```python
from build123d import *

# Parameters (mm, degrees)
BOSS_EXTRUDE1_DEPTH       = 45
M6X1_0_TAPPED_HOLE1_D     = 5
M6X1_0_TAPPED_HOLE1_DEPTH = 10
M6X1_0_TAPPED_HOLE1_TIP   = 1.502151548
SKETCH5_R                 = 12.5
SKETCH5_R_2               = 14.5
CUT_EXTRUDE1_DEPTH        = 10
SKETCH6_R                 = 14.5
CUT_EXTRUDE2_DEPTH        = 3
CUT_EXTRUDE3_DEPTH        = 86.755466298
CUT_EXTRUDE3_DEPTH_BACK   = 86.755466298
SKETCH7_R                 = 8
CIRPATTERN1_COUNT         = 8


with BuildPart() as part:
    # Sketch1 → Boss-Extrude1 (new body)
    with BuildSketch(Plane.XY):
        Polygon((-45.5, 0), (45.5, 0), (55, 9.5), (55, 48), (45, 48), (45, 39), (-45, 39), (-45, 48), (-55, 48), (-55, 9.5), align=None)
    extrude(amount=BOSS_EXTRUDE1_DEPTH)

    # M6x1.0 Tapped Hole1
    with Locations(Plane(origin=(0, 48, 0), x_dir=(1, 0, 0), z_dir=(0, 1, 0))):
        with Locations((-50, -7.5), (50, -7.5), (50, -37.5), (-50, -37.5)):
            Hole(M6X1_0_TAPPED_HOLE1_D / 2, depth=M6X1_0_TAPPED_HOLE1_DEPTH)
            with Locations((0, 0, -(M6X1_0_TAPPED_HOLE1_DEPTH + M6X1_0_TAPPED_HOLE1_TIP / 2))):  # 118° drill point
                Cone(0, M6X1_0_TAPPED_HOLE1_D / 2, M6X1_0_TAPPED_HOLE1_TIP, mode=Mode.SUBTRACT)

    # Sketch5 → Cut-Extrude1 (cut)
    with BuildSketch(Plane.XY.offset(45)):
        with Locations((-35, 19.5)):
            Circle(SKETCH5_R)
        with Locations((0, 19.5)):
            Circle(SKETCH5_R_2)
        with Locations((35, 19.5)):
            Circle(SKETCH5_R)
    extrude(amount=-CUT_EXTRUDE1_DEPTH, mode=Mode.SUBTRACT)

    # Sketch6 → Cut-Extrude2 (cut)
    with BuildSketch(Plane.XY.offset(35)):
        with Locations((0, 19.5)):
            Circle(SKETCH6_R)
    extrude(amount=-CUT_EXTRUDE2_DEPTH, mode=Mode.SUBTRACT)

    # Sketch7 → Cut-Extrude3 (cut, two sides: drawn at the far end of the back side and taken through both)
    with BuildSketch(Plane.XY.offset(-CUT_EXTRUDE3_DEPTH_BACK)):
        with Locations((0, 19.5)):
            Circle(SKETCH7_R)
        with Locations((35, 19.5)):
            Circle(SKETCH7_R)
        with Locations((-35, 19.5)):
            Circle(SKETCH7_R)
    extrude(amount=CUT_EXTRUDE3_DEPTH + CUT_EXTRUDE3_DEPTH_BACK, mode=Mode.SUBTRACT)

    # Sketch11 → M6x1.0 Tapped Hole2 (revolve, cut)
    with BuildSketch(Plane(origin=(19, 19.5, 0), x_dir=(0, 1, 0), z_dir=(1, 0, 0))):
        Polygon((0, 0), (0, 16.502151548), (2.5, 15), (2.5, 0), align=None)
    m6x1_0_tapped_hole2 = revolve(axis=Axis((19, 19.5, -6.35), (0, 0, 1)), mode=Mode.SUBTRACT)

    # CirPattern1: M6x1.0 Tapped Hole2 ×8 about axis, 2 skipped
    cirpattern1_axis = Axis((0, 19.5, 0), (0, 0, -1))
    add([m6x1_0_tapped_hole2.rotate(cirpattern1_axis, i * 360 / CIRPATTERN1_COUNT) for i in range(1, CIRPATTERN1_COUNT) if i not in (2, 6)], mode=Mode.SUBTRACT)


solid = part.part
```
Source: CAD feature listing. Evaluate the final solid. Frame: model axes, mm. A direction names the side the tool comes from. Round coordinates to 2 decimals unless told otherwise and drop trailing zeros. Loops run counter-clockwise (first coordinate to the right, second up) from the corner with the lowest first, then second, coordinate; pieces in that order, holes last. Notation, with made-up numbers: M 38.25,-2 L 94.25,-2 A19 ccw 94.25,24 Z; hole C 82.25,86 d11. An arc over 180 degrees is marked long. Use a Markdown table: item, result. Add a question column.
1. Line query: line 1 (X direction, y = 19, z = 19); line 2 (Z direction, x = 50, y = 41); line 3 (X direction, y = 19, z = 33). Output: solid intervals per line, ascending.
2. Section query A-A on x = -35. Return the cut outline in (y, z), then the cut area to 3 significant figures.
3. Contact query for flat-ended pins moving along their axis: P1, Ø1.5, axis at x = 2, z = 23, coming from the -Y side; P2, Ø6, axis at x = -50, z = 7.5, coming from the -Y side; P3, Ø3, axis at x = -50, z = 37.5, coming from the +Y side; P4, Ø13.5, axis at x = 12, z = 23, coming from the +Y side. Output: stop coordinate, or through.
4. Section query B-B on z = 12. Give the number of separate pieces and of enclosed holes in the cut face, then the cut area to 3 significant figures.
5. Section query C-C on y = 14.5. Return the cut outline in (x, z) (3 decimals), then the cut area to 3 significant figures.
6. Mould query, pull axis Y, two halves, no side actions, for faces 6 (the flat face through (6, 13, 32)), 7 (the conical face through (50.4, 36.76, 37.67)), 8 (the cylindrical face through (-52.31, 42.93, 8.46)). Classes: pulls with the +Y half, pulls with the -Y half, needs draft (parallel to the pull), parting line crosses it, or undercut.
7. Section query D-D on x = 39.5. Return the cut outline in (y, z), then the cut area to 3 significant figures.
8. Reachability of faces 1 (the flat face through (-55, 29, 22)), 2 (the cylindrical face through (12.895, 8.506, 7.395)), 3 (the cylindrical face through (47.69, 42.93, 38.46)), 4 (the flat face through (45, 44, 22)), 5 (the flat face through (35, 11, 35)) from +Z, -Z, +X, -X, +Y, -Y: full face, straight path, thin tool, end or side. Return the list, or none.
Reported:
| question | item | result |
|---|---|---|
| 1 | line 1 | x = -55 to -42.98, -27.02 to -7.98, 7.98 to 27.02, 42.98 to 55 |
| 1 | line 2 | z = 0 to 5, 10 to 35, 40 to 45 |
| 1 | line 3 | x = -55 to -42.98, -27.02 to -14.49, 14.49 to 27.02, 42.98 to 55 |
| 2 | outline | M 0,0 L 11.5,0 L 11.5,35 L 7,35 L 7,45 L 0,45 Z; M 27.5,0 L 39,0 L 39,45 L 32,45 L 32,35 L 27.5,35 Z |
| 2 | area | 945 mm² |
| 3 | P1 | stops at y = 0 |
| 3 | P2 | stops at y = 1.5 |
| 3 | P3 | stops at y = 37.4 |
| 3 | P4 | stops at y = 39 |
| 4 | separate pieces | 1 |
| 4 | enclosed holes | 9 |
| 4 | area | 3,660 mm² |
| 5 | outline | M -55,0 L -41.245,0 L -41.245,35 L -46.456,35 L -46.456,45 L -55,45 Z; M -28.755,0 L -6.245,0 L -6.245,32 L -13.611,32 L -13.611,45 L -23.544,45 L -23.544,35 L -28.755,35 Z; M 6.245,0 L 28.755,0 L 28.755,35 L 23.544,35 L 23.544,45 L 13.611,45 L 13.611,32 L 6.245,32 Z; M 41.245,0 L 55,0 L 55,45 L 46.456,45 L 46.456,35 L 41.245,35 Z |
| 5 | area | 2,860 mm² |
| 6 | face 6 | undercut |
| 6 | face 7 | pulls with the +Y half |
| 6 | face 8 | needs draft |
| 7 | outline | M 0,0 L 12.89,0 L 12.89,35 L 7.84,35 L 7.84,45 L 0,45 Z; M 26.11,0 L 39,0 L 39,45 L 31.16,45 L 31.16,35 L 26.11,35 Z |
| 7 | area | 1,060 mm² |
| 8 | face 1 | +Z, -Z, -X, +Y, -Y |
| 8 | face 2 | -Z |
| 8 | face 3 | +Y |
| 8 | face 4 | +Z, -Z, +Y |
| 8 | face 5 | +Z |
